Can you work these out from the model? Positions are in its coordinate system, mm. Round coordinates to 2 decimals unless told otherwise and drop trailing zeros. Order: outer loops, then holes, each group sorted by start corner. A loop starts at its lowest first (then second) coordinate and runs counter-clockwise, first axis right, second up.
from build123d import *
from build123d.topology import SkipClean

# Parameters (mm, degrees)
SKETCH_1_R      = 4
SKETCH_1_R_2    = 1.6
EXTRUDE_1_DEPTH = 8
EXTRUDE_START   = 2
SKETCH_2_R      = 1.6
EXTRUDE_2_DEPTH = 2


with BuildPart() as part:
    # Эскиз1 → Бобышка-Вытянуть1 (new body)
    with BuildSketch(Plane.XY):
        Circle(SKETCH_1_R)
        Circle(SKETCH_1_R_2, mode=Mode.SUBTRACT)
    extrude(amount=EXTRUDE_1_DEPTH)

    # Эскиз2 → Бобышка-Вытянуть2 (add)
    with SkipClean():  # the faces are left unmerged after this step: merging them gives an invalid solid
        with BuildSketch(Plane(origin=(0, 0, 0), x_dir=(-1, 0, 0), z_dir=(0, 0, -1)).offset(EXTRUDE_START)):
            with BuildLine():
                Line((0, -4), (12.370366619, -4))
                ThreePointArc((12.370366619, -4), (16.017109836, 0), (12.370366619, 4))
                Line((12.370366619, 4), (0, 4))
                ThreePointArc((0, 4), (-4, 0), (0, -4))
            make_face()
            with Locations((12, 0)):
                Circle(SKETCH_2_R, mode=Mode.SUBTRACT)
            Circle(SKETCH_2_R, mode=Mode.SUBTRACT)
        extrude(amount=-EXTRUDE_2_DEPTH)


solid = part.part
(1) I want a section at A-A, the plane y = 0. List the corners of the cut face in (x, z) for me, plus the area to 3 significant figures.
(2) I want a section at D-D, the plane x = -2. List the corners of the cut face in (y, z) for me, plus the area to 3 significant figures.
(3) I want a section at C-C, the plane z = 0.5. List the corners of the cut face in (x, y) for me.
(4) Please list where these lines run through material, in increasing order: probe 1 along Y at (x, z) = (-12, -1.45); probe 2 along Z at (x, y) = (-14, 1.5).
(5) I'm going to push flat-ended pins straight in: pin 1 Ø2.5 at (x, y) = (-8, -0.5) entering from +Z; pin 2 Ø1.9 at (x, y) = (0, 0) entering from +Z; pin 3 Ø2 at (y, z) = (1.5, 4.5) entering from +X; pin 4 Ø4 at (x, z) = (0.5, 2.5) entering from +Y. Where does each tip first touch, or does it pass through?
(6) If we mould it in two halves opening along X, with no side actions, what happens to faces 1 (the face through (-16.016, -0.083, -1.014)), 2 (the face through (-10.4, 0.07, -1.01)), 3 (the face through (-10, 0, 0))? For each: pulls with the +X half, pulls with the -X half, needs draft (parallel to the pull), parting line crosses it, or undercut.
(7) I want a section at B-B, the plane x = -12. List the corners of the cut face in (y, z) for me.
Ans:
1. outline: (-16.02, -2) - (-13.6, -2) - (-13.6, 0) - (-16.02, 0) - close; (-10.4, -2) - (-1.6, -2) - (-1.6, 8) - (-4, 8) - (-4, 0) - (-10.4, 0) - close; (1.6, -2) - (4, -2) - (4, 8) - (1.6, 8) - close
1. area: 65.6 mm2
2. outline: (-4, -2) - (4, -2) - (4, 0) - (3.46, 0) - (3.46, 8) - (-3.46, 8) - (-3.46, 0) - (-4, 0) - close
2. area: 71.4 mm2
3. outline: circle Ø8 at (0, 0); hole circle Ø3.2 at (0, 0)
4. probe 1: y = -4 to -1.6, 1.6 to 4
4. probe 2: z = -2 to 0
5. pin 1: stops at z = 0
5. pin 2: passes through
5. pin 3: stops at x = 3.97
5. pin 4: stops at y = 4
6. face 1: pulls with the -X half
6. face 2: undercut
6. face 3: needs draft
7. outline: (-4, -2) - (-1.6, -2) - (-1.6, 0) - (-4, 0) - close; (1.6, -2) - (4, -2) - (4, 0) - (1.6, 0) - close
